Here's how the part is built. I have some questions about the finished solid (model axes, mm). A direction names the side the tool comes from. Give positions to 0.01 mm unless a question says otherwise; leave off trailing zeros. Write each loop counter-clockwise with the first axis right and the second up, starting at its lowest first coordinate (ties: lowest second). Pieces come first, ordered by that corner, then holes. Notation, with made-up numbers: (60.5, 48) -> (91.5, 48) arc R28 ccw to (91.5, 83) -> close; hole circle Ø8 at (19.25, 65). An arc over 180 degrees is marked (long way). Answer as CSV lines item,"result". Start each with the question number.
from build123d import *

# Parameters (mm, degrees)
SKETCH_1_R      = 1.525
SKETCH_1_W      = 41.5
SKETCH_1_H      = 21.5
SKETCH_1_W_2    = 10
SKETCH_1_H_2    = 3
EXTRUDE_1_DEPTH = 3


with BuildPart() as part:
    # 草图1 → 凸台-拉伸1 (new body)
    with BuildSketch(Plane(origin=(0, 0, 0), x_dir=(1, 0, 0), z_dir=(0, 1, 0))):
        Polygon((15, 10), (-15, 10), (-24.93, 15.75), (-77.43, 15.75), (-82.43, 10.75), (-82.43, -10.75), (-77.43, -15.75), (-24.93, -15.75), (-15, -10), (15, -10), (24.93, -15.75), (77.43, -15.75), (82.43, -10.75), (82.43, 10.75), (77.43, 15.75), (24.93, 15.75), align=None)
        with Locations(Location((-77.98, 4.875, 0), (0, 0, 270))):
            Circle(SKETCH_1_R, mode=Mode.SUBTRACT)
        with Locations(Location((-77.98, -4.875, 0), (0, 0, 90))):
            Circle(SKETCH_1_R, mode=Mode.SUBTRACT)
        with Locations(Location((77.98, -4.875, 0), (0, 0, 270))):
            Circle(SKETCH_1_R, mode=Mode.SUBTRACT)
        with Locations(Location((77.98, 4.875, 0), (0, 0, 90))):
            Circle(SKETCH_1_R, mode=Mode.SUBTRACT)
        with Locations(Location((-29.38, 4.875, 0), (0, 0, 270))):
            Circle(SKETCH_1_R, mode=Mode.SUBTRACT)
        with Locations(Location((-29.38, -4.875, 0), (0, 0, 90))):
            Circle(SKETCH_1_R, mode=Mode.SUBTRACT)
        with Locations(Location((29.38, -4.875, 0), (0, 0, 270))):
            Circle(SKETCH_1_R, mode=Mode.SUBTRACT)
        with Locations(Location((29.38, 4.875, 0), (0, 0, 90))):
            Circle(SKETCH_1_R, mode=Mode.SUBTRACT)
        with Locations((-53.68, 0)):
            Rectangle(SKETCH_1_W, SKETCH_1_H, mode=Mode.SUBTRACT)
        with Locations((-15, 0)):
            Rectangle(SKETCH_1_W_2, SKETCH_1_H_2, mode=Mode.SUBTRACT)
        with Locations((53.68, 0)):
            Rectangle(SKETCH_1_W, SKETCH_1_H, mode=Mode.SUBTRACT)
        with Locations((15, 0)):
            Rectangle(SKETCH_1_W_2, SKETCH_1_H_2, mode=Mode.SUBTRACT)
    extrude(amount=EXTRUDE_1_DEPTH)


solid = part.part
Item 1: If we section it at D-D (y = 1.75): State how many separate pieces and enclosed holes the cut face has, and give its area (3 significant figures).
Item 2: If we section it at B-B (x = 12): Please give me the cut outline in (y, z).
Item 3: If we section it at A-A (x = -29.38): Please give me the cut outline in (y, z), and give its area (3 significant figures).
Item 4: We'd pull the mould along Z, two halves only. Please class faces 4 (the face through (-15, 1, 1.5)), 5 (the face through (-79.96, 1.48, 13.22)), 6 (the face through (-51, 1, -15.75)): released by +Z, released by -Z, zero draft, split by the parting line, or undercut.
Item 5: For faces 1 (the face through (-79.9, 1.48, -13.28)), 2 (the face through (10, 1, 0)), 3 (the face through (20.035, 1.479, -12.915)), which set-ups out of +Z, -Z, +X, -X, +Y, -Y let a thin tool reach every point of the face, with its end or its side?
Item 6: If I drill on line 1 (X direction, y = 1.3, z = 1); line 2 (X direction, y = 0.55, z = 9); line 3 (Z direction, x = 43, y = 2.2), over which ranges is the centre line in solid material (lowest first)? Write a range as [from, to].
Item 7: I'm going to push a flat-ended pin straight in: pin 1 (0.9 mm diameter, centred on x = 3, y = 1, fed in from +Z). Where does the tip first touch, or does it pass through?
Item 8: If we section it at C-C (z = -14): Please give me the cut outline in (x, y).
Final values:
1,separate pieces,"1"
1,enclosed holes,"12"
1,area,"2,780 mm2"
2,outline,"(0, -10) -> (3, -10) -> (3, -1.5) -> (0, -1.5) -> close; (0, 1.5) -> (3, 1.5) -> (3, 10) -> (0, 10) -> close"
3,outline,"(0, -15.75) -> (3, -15.75) -> (3, -6.4) -> (0, -6.4) -> close; (0, -3.35) -> (3, -3.35) -> (3, 3.35) -> (0, 3.35) -> close; (0, 6.4) -> (3, 6.4) -> (3, 15.75) -> (0, 15.75) -> close"
3,area,"76.2 mm2"
4,face 4,"undercut"
4,face 5,"released by +Z"
4,face 6,"released by -Z"
5,face 1,"-Z, -X, +Y, -Y"
5,face 2,"+Y, -Y"
5,face 3,"-Z, +Y, -Y"
6,line 1,"[-82.43, -74.43], [-32.93, -20], [-10, 10], [20, 32.93], [74.43, 82.43]"
6,line 2,"[-82.43, -74.43], [-32.93, 32.93], [74.43, 82.43]"
6,line 3,"[-15.75, -10.75], [10.75, 15.75]"
7,pin 1,"z = 10"
8,outline,"(-79.18, 0) -> (-21.91, 0) -> (-21.91, 3) -> (-79.18, 3) -> close; (21.91, 0) -> (79.18, 0) -> (79.18, 3) -> (21.91, 3) -> close"
